The listing builds one solid part. Answer for the finished solid, in the listing's coordinates (mm). A direction names the side the tool comes from. Coordinates: 2 decimals unless noted, no trailing zeros. Order: outer loops, then holes, each group sorted by start corner. A loop starts at its lowest first (then second) coordinate and runs counter-clockwise, first axis right, second up. Notation, with made-up numbers: (83, -11.75) -> (130, -11.75) arc R15 ccw to (130, 10.25) -> close; hole circle Ø4 at (52, 14). An arc over 180 degrees is marked (long way). Put each result on its own line as item: value. Start each with the question number.
Autodesk Inventor part; units mm, degrees
ref_plane "YZ Plane" through (0, 0, 0) normal (1, 0, 0) x (0, 1, 0)
ref_plane "XZ Plane" through (0, 0, 0) normal (0, 1, 0) x (-1, 0, 0)
ref_plane "XY Plane" through (0, 0, 0) normal (0, 0, 1) x (1, 0, 0)
sketch "Sketch1" plane through (0, 0, 0) normal (1, 0, 0) x (0, 1, 0)
  circle A0 centre (0, 0) radius 31.5
  dimension "d0" = 63
extrude "Extrusion1" add sketch "Sketch1" along normal blind 75
sketch "Sketch2" plane through (75, 0, 0) normal (1, 0, 0) x (0, 0, -1)
  circle A0 centre (0, 0) radius 4
  dimension "d3" = 8
extrude "Extrusion2" add sketch "Sketch2" along normal blind 24
sketch "Sketch3" plane through (75, 0, 0) normal (1, 0, 0) x (0, 0, -1)
  circle A0 centre (0, 15) radius 2
  circle A1 centre (0, 22) radius 2
  circle A2 centre (15, 0) radius 2
  circle A3 centre (22, 0) radius 2
  circle A4 centre (0, -15) radius 2
  circle A5 centre (0, -22) radius 2
  circle A6 centre (-15, 0) radius 2
  circle A7 centre (-22, 0) radius 2
  point P0 (0, 0)
  dimension "d8" = 4
  dimension "d9" = 4
  dimension "d10" = 4
  dimension "d11" = 4
  dimension "d12" = 4
  dimension "d13" = 4
  dimension "d14" = 4
  dimension "d15" = 4
extrude "Extrusion3" cut sketch "Sketch3" against normal blind 8
sketch "Sketch4" plane through (0, 0, 0) normal (-1, 0, 0) x (0, 0, 1)
  circle A0 centre (0, 0) radius 4
  circle A1 centre (0, 0) radius 31.5
extrude "Extrusion4" cut sketch "Sketch4" against normal blind 20 contours A0 | A1
sketch "Sketch5" plane through (75, 0, 0) normal (1, 0, 0) x (0, 0, -1)
  arc A0 (22.2739, -22.2739) -> (-22.2739, -22.2739) centre (0, 0) ccw
  arc A1 (17.3205, -10) -> (-17.3205, -10) centre (0, 0) ccw
  arc A2 (11.2583, -6.5) -> (-11.2583, -6.5) centre (0, 0) ccw
  arc A3 (14.7224, -8.5) -> (-14.7224, -8.5) centre (0, 0) ccw
  arc A4 (20.7846, -12) -> (-20.7846, -12) centre (0, 0) ccw
  line L0 (0, 0) -> (31.5, 0) construction
  arc A5 (-20.7846, -12) -> (-17.3205, -10) centre (-19.0526, -11) ccw
  arc A6 (-14.7224, -8.5) -> (-11.2583, -6.5) centre (-12.9904, -7.5) ccw
  arc A7 (11.2583, -6.5) -> (14.7224, -8.5) centre (12.9904, -7.5) ccw
  arc A8 (17.3205, -10) -> (20.7846, -12) centre (19.0526, -11) ccw
  line L1 (0, 0) -> (31.5, 0) construction
  line L2 (0, 0) -> (-2.8284, -2.8284)
  line L3 (-9.1924, -9.1924) -> (-22.2739, -22.2739)
  line L4 (9.1924, -9.1924) -> (22.2739, -22.2739)
  arc A9 (-9.1924, -9.1924) -> (9.1924, -9.1924) centre (0, 0) ccw
  arc A10 (11.2583, -6.5) -> (-11.2583, -6.5) centre (0, 0) ccw
  circle A11 centre (0, 0) radius 5
  dimension "d23" = 10
properties part number "MotorModel"
(1) The part is cut by section D-D on x = 33. Determine the outline of the cut face in (y, z), plus the area to 3 significant figures.
(2) Find the intervals of material crossed by L1, parallel to X at y = -1.5, z = -24; L2, parallel to X at y = 23, z = -1.5; L3, parallel to Y at x = 70, z = 15, in increasing order.
(3) The part is cut by section B-B on y = -22. Determine the outline of the cut face in (x, z).
(4) For a pull along Z with two mould halves and no side action, classify faces 3 (the cylindrical face through (86.832, 3.905, 0.867)), 4 (the cylindrical face through (71, -20, 0)), 5 (the flat face through (75, 7, 0)) as released by +Z, released by -Z, zero draft, split by the parting line, or undercut.
(5) The part is cut by section A-A on z = 15. Determine the outline of the cut face in (x, y), plus the area to 3 significant figures.
(6) The part is cut by section C-C on x = 84. Determine the outline of the cut face in (y, z).
(7) Each of these flat-tipped pins is pushed along its axis until it touches: P1, Ø2, axis at x = 73, z = 5, coming from the +Y side (3 decimals); P2, Ø3, axis at y = 22, z = 0, coming from the +X side; P3, Ø5, axis at x = 56.5, y = -8, coming from the -Z side; P4, Ø4, axis at x = 90, z = -7.5, coming from the -Y side. Where does it stop, or does it pass through?
(8) A tool of negligible diameter and unlimited length cuts with its end or side. For faces 1 (the flat face through (20, 0, 0)), 2 (the cylindrical face through (71.1, -1.2, 16.6)), from which of +Z, -Z, +X, -X, +Y, -Y can it reach the whole face along a straight path? Write none if from no direction.
Worked out:
1. outline: circle Ø63 at (0, 0)
1. area: 3,120 mm2
2. L1: 20 to 75
2. L2: 20 to 67
2. L3: -27.7 to -2, 2 to 27.7
3. outline: (20, -22.54) -> (75, -22.54) -> (75, -2) -> (67, -2) -> (67, 2) -> (75, 2) -> (75, 22.54) -> (20, 22.54) -> close
4. face 3: split by the parting line
4. face 4: undercut
4. face 5: zero draft
5. outline: (20, -27.7) -> (75, -27.7) -> (75, -2) -> (67, -2) -> (67, 2) -> (75, 2) -> (75, 27.7) -> (20, 27.7) -> close
5. area: 3,010 mm2
6. outline: circle Ø8 at (0, 0)
7. P1: y = 31.245
7. P2: x = 67
7. P3: z = -31.02
7. P4: through
8. face 1: +Z, -Z, -X, +Y, -Y
8. face 2: +X
